Geometry check sheet. Reference: the model listing, model coordinates, mm. Face numbers are marked on the shaded views. Round coordinates to 2 decimals unless told otherwise and drop trailing zeros. Write each loop counter-clockwise with the first axis right and the second up, starting at its lowest first coordinate (ties: lowest second). Pieces come first, ordered by that corner, then holes.
from build123d import *

# Parameters (mm, degrees)
SKETCH_1_W          = 52
SKETCH_1_H          = 52.00000000000001
SKETCH_1_W_2        = 32
SKETCH_1_H_2        = 32
SKETCH_1_R          = 1.6000000000000019
EXTRUDE_2_DEPTH     = 20
SHELL_6_T           = -2
SKETCH_3_W          = 52
SKETCH_3_H          = 52.00000000000001
SKETCH_3_W_2        = 50
SKETCH_3_H_2        = 50.00000000000001
CUT_EXTRUDE_5_DEPTH = 4
CUT_EXTRUDE_6_DEPTH = 62.4817045957576
CUT_EXTRUDE_7_DEPTH = 62.48170459575759


with BuildPart() as part:
    # 草图1 → 凸台-拉伸2 (new body)
    # profile 1 of 2: a face of its own
    with BuildSketch(Plane(origin=(0, 0, 0), x_dir=(1, 0, 0), z_dir=(0, 1, 0))):
        Rectangle(SKETCH_1_W, SKETCH_1_H)
        Rectangle(SKETCH_1_W_2, SKETCH_1_H_2, mode=Mode.SUBTRACT)
    # profile 2 of 2: a face of its own
    with BuildSketch(Plane(origin=(0, 0, 0), x_dir=(1, 0, 0), z_dir=(0, 1, 0))):
        Rectangle(SKETCH_1_W_2, SKETCH_1_H_2)
        with Locations(Location((-13.000000000000002, -13.000000000000002, 0), (0, 0, 270))):
            Circle(SKETCH_1_R, mode=Mode.SUBTRACT)
        with Locations(Location((13.000000000000009, -13.000000000000002, 0), (0, 0, 270))):
            Circle(SKETCH_1_R, mode=Mode.SUBTRACT)
        with Locations(Location((-13.000000000000002, 13.000000000000002, 0), (0, 0, 270))):
            Circle(SKETCH_1_R, mode=Mode.SUBTRACT)
        with BuildLine():
            Line((-7.599999999999996, -7.550000000000001), (-7.599999999999996, -1.9999999999999991))
            Line((-7.599999999999996, -1.9999999999999991), (-11.599999999999998, -1.9999999999999996))
            ThreePointArc((-11.599999999999998, -1.9999999999999996), (-13.599999999999998, 2.4e-16), (-11.599999999999998, 1.9999999999999996))
            Line((-11.599999999999998, 1.9999999999999996), (-7.599999999999996, 1.9999999999999991))
            Line((-7.599999999999996, 2), (-7.599999999999996, 7.549999999999999))
            Line((-7.599999999999996, 7.549999999999999), (7.600000000000003, 7.549999999999999))
            Line((7.600000000000004, 7.549999999999999), (7.600000000000004, 2))
            Line((7.600000000000002, 1.9999999999999991), (11.600000000000005, 1.9999999999999996))
            ThreePointArc((11.600000000000005, 1.9999999999999996), (13.0142135623731, 1.4142135623730947), (13.600000000000005, 0))
            ThreePointArc((13.600000000000005, -4.9e-16), (13.014213562373099, -1.4142135623730951), (11.600000000000005, -1.9999999999999996))
            Line((11.600000000000005, -1.9999999999999996), (7.600000000000002, -1.9999999999999991))
            Line((7.600000000000004, -1.9999999999999991), (7.600000000000004, -7.550000000000001))
            Line((7.600000000000003, -7.550000000000001), (-7.599999999999996, -7.550000000000001))
        make_face(mode=Mode.SUBTRACT)
        with Locations(Location((13.000000000000009, 13.000000000000002, 0), (0, 0, 270))):
            Circle(SKETCH_1_R, mode=Mode.SUBTRACT)
    extrude(amount=EXTRUDE_2_DEPTH)

    # 抽壳6
    shell_6_openings = [part.faces().sort_by_distance(p)[0] for p in [
        (-25.264608948, 20, 0),
        (-13, 10, 11.4),
        (13, 10, 11.4),
        (7.6, 10, -4.775),
        (0, 10, -7.55),
        (-7.6, 10, -4.775),
        (-9.6, 10, -2),
        (-13.6, 10, 0),
        (-9.6, 10, 2),
        (-7.6, 10, 4.775),
        (0, 10, 7.55),
        (7.6, 10, 4.775),
        (9.6, 10, 2),
        (13.6, 10, 0),
        (9.6, 10, -2),
        (-13, 10, -14.6),
        (13, 10, -14.6),
    ]]
    offset(amount=SHELL_6_T, openings=shell_6_openings, kind=Kind.INTERSECTION)

    # 草图3 → 切除-拉伸5 (cut)
    with BuildSketch(Plane(origin=(0, 20, 0), x_dir=(1, 0, 0), z_dir=(0, 1, 0))):
        Rectangle(SKETCH_3_W, SKETCH_3_H)
        Rectangle(SKETCH_3_W_2, SKETCH_3_H_2, mode=Mode.SUBTRACT)
    extrude(amount=-CUT_EXTRUDE_5_DEPTH, mode=Mode.SUBTRACT)

    # 草图4 → 切除-拉伸6 (cut, through all)
    with BuildSketch(Plane.XY.offset(26.000000000000004)):
        Polygon((22.499999999999993, 3.0000000000000044), (-22.500000000000007, 2.999999999999999), (-22.500000000000007, 13), (22.499999999999993, 13.000000000000007), align=None)
    extrude(amount=-CUT_EXTRUDE_6_DEPTH, mode=Mode.SUBTRACT)

    # 草图5 → 切除-拉伸7 (cut, through all)
    with BuildSketch(Plane.ZY.offset(25.999999999999996)):
        Polygon((0, 8), (0, 13), (-22.500000000000007, 12.999999999999996), (-22.500000000000007, 8), align=None)
        Polygon((22.499999999999993, 13.000000000000004), (0, 13), (0, 8), (22.499999999999996, 8), align=None)
        Polygon((22.499999999999996, 8), (0, 8), (0, 2.9999999999999982), (22.499999999999993, 3.000000000000001), align=None)
        Polygon((0, 2.9999999999999982), (0, 8), (-22.500000000000007, 8), (-22.500000000000007, 2.9999999999999956), align=None)
    extrude(amount=-CUT_EXTRUDE_7_DEPTH, mode=Mode.SUBTRACT)


solid = part.part
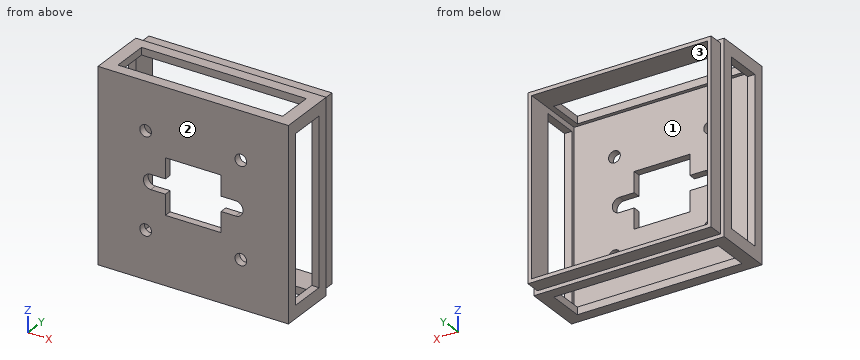
1. Section check D-D (z = 3.5). Record the cut outline in (x, y), plus the area to 3 significant figures.
2. Scan lines: line 1 along X through (y, z) = (1.05, 13); line 2 along X through (y, z) = (18, -12.5); line 3 along X through (y, z) = (2.25, 0). Record each from-to range of solid material in increasing order.
3. Section check B-B (x = 21). Record the cut outline in (y, z), plus the area to 3 significant figures.
4. Release check for a two-part mould opening along X. For the marked faces 1, 2 and 3 record: +X half, -X half, draft (parallel to the pull), parting line (faces both ways), or undercut.
5. Section check C-C (z = -13). Record the cut outline in (x, y), plus the area to 3 significant figures.
6. Section check A-A (z = 19.5). Record the cut outline in (x, y), plus the area to 3 significant figures.
7. Depth check by flat-ended pin: pin 1 Ø1.2 at (y, z) = (18, 12.5) entering from -X; pin 2 Ø1.6 at (x, z) = (-1.5, 25) entering from -Y; pin 3 Ø1 at (x, z) = (-3, -20) entering from +Y; pin 4 Ø1.2 at (x, y) = (-2.5, 18.5) entering from +Z. Enter the tip coordinate at first touch or a pass-through.
Results below:
1. outline: (-26, 0) - (-7.6, 0) - (-7.6, 2) - (-24, 2) - (-24, 3) - (-26, 3) - close; (-26, 13) - (-24, 13) - (-24, 20) - (-25, 20) - (-25, 16) - (-26, 16) - close; (7.6, 0) - (26, 0) - (26, 3) - (24, 3) - (24, 2) - (7.6, 2) - close; (24, 13) - (26, 13) - (26, 16) - (25, 16) - (25, 20) - (24, 20) - close
1. area: 97.6 mm2
2. line 1: x = -26 to -14.6, -11.4 to 11.4, 14.6 to 26
2. line 2: x = -25 to -24, 24 to 25
2. line 3: x = -26 to -24, 24 to 26
3. outline: (0, -26) - (3, -26) - (3, -24) - (2, -24) - (2, 24) - (3, 24) - (3, 26) - (0, 26) - close; (13, -26) - (16, -26) - (16, -25) - (20, -25) - (20, -24) - (13, -24) - close; (13, 24) - (20, 24) - (20, 25) - (16, 25) - (16, 26) - (13, 26) - close
3. area: 128 mm2
4. face 1: undercut
4. face 2: draft
4. face 3: undercut
5. outline: (-26, 0) - (-14.6, 0) - (-14.6, 2) - (-24, 2) - (-24, 3) - (-26, 3) - close; (-26, 13) - (-24, 13) - (-24, 20) - (-25, 20) - (-25, 16) - (-26, 16) - close; (-11.4, 0) - (11.4, 0) - (11.4, 2) - (-11.4, 2) - close; (14.6, 0) - (26, 0) - (26, 3) - (24, 3) - (24, 2) - (14.6, 2) - close; (24, 13) - (26, 13) - (26, 16) - (25, 16) - (25, 20) - (24, 20) - close
5. area: 115 mm2
6. outline: (-26, 0) - (26, 0) - (26, 3) - (24, 3) - (24, 2) - (-24, 2) - (-24, 3) - (-26, 3) - close; (-26, 13) - (-24, 13) - (-24, 20) - (-25, 20) - (-25, 16) - (-26, 16) - close; (24, 13) - (26, 13) - (26, 16) - (25, 16) - (25, 20) - (24, 20) - close
6. area: 128 mm2
7. pin 1: stops at x = -25
7. pin 2: stops at y = 0
7. pin 3: stops at y = 2
7. pin 4: stops at z = 25
